Part print with two shaded views. Sizes in mm from the minimum x, y, z corner. A direction names the side the tool comes from. Round coordinates to 2 decimals unless told otherwise and drop trailing zeros. Order: outer loops, then holes, each group sorted by start corner. A loop starts at its lowest first (then second) coordinate and runs counter-clockwise, first axis right, second up. Notation, with made-up numbers: (46, -35.75) -> (53, -35.75) arc R32 ccw to (53, -5.75) -> close; hole circle Ø4 at (4, -14.75). An arc over 180 degrees is marked (long way). Put each result on its own line as item: value. Start each with the question number.
Q1. 3-axis set-ups, long thin cutter, end or side, ignore diameter. For the marked faces 4 and 5: which of +Z, -Z, +X, -X, +Y, -Y reach the whole face in a straight line?
Q2. Flat gauge pins, fed straight in: P1, Ø8, axis at x = 15.5, z = 28.5, coming from the +Y side; P2, Ø4.5, axis at y = 45, z = 10.5, coming from the -X side; P3, Ø20, axis at x = 40.5, y = 28, coming from the -Z side; P4, Ø1.9, axis at x = 29.19, y = 17.25, coming from the -Z side. Where does each tip first touch, or does it go through?
Q3. Probe L1, parallel to X at y = 47, z = 10; L2, parallel to Y at x = 61, z = 7; L3, parallel to Y at x = 17.5, z = 31.95. List the from-to ranges inside material, lowest first.
Q4. Pull direction Y, two halves, no side cores. Call the marked faces 1, 2 and 3: released by +Y, released by -Y, zero draft, split by the parting line, or undercut.
Q5. Cut at D-D, the plane y = 26. List the corners of the cut face in (x, z) (1 decimal).
Q6. Cut at B-B, the plane x = 92.5. List the corners of the cut face in (y, z), and give its area (3 significant figures).
Q7. Cut at A-A, the plane z = 15. List the corners of the cut face in (x, y).
Q8. Cut at C-C, the plane x = 81. List the corners of the cut face in (y, z).
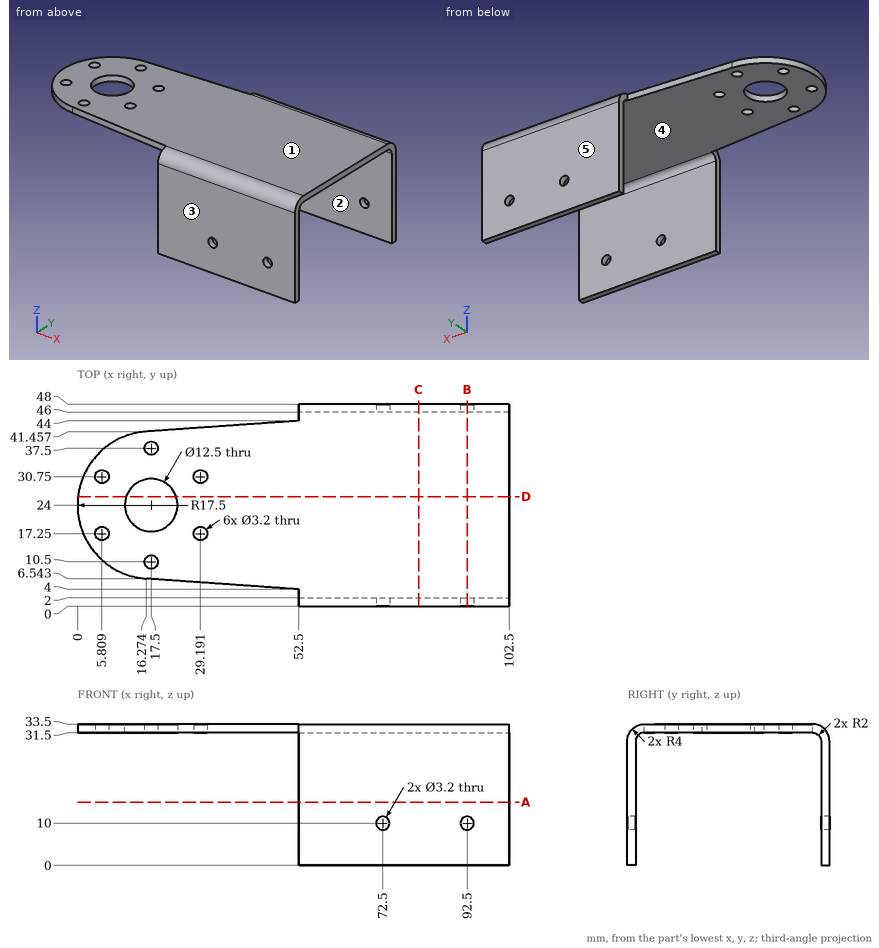
Ans:
1. face 4: -Z, +X, -X
1. face 5: +Z, -Z, +X, -X, +Y
2. P1: stops at y = 41.59
2. P2: stops at x = 52.5
2. P3: stops at z = 31.5
2. P4: passes through
3. L1: x = 52.5 to 70.9, 74.1 to 90.9, 94.1 to 102.5
3. L2: y = 0 to 2, 46 to 48
3. L3: y = 6.46 to 8.9, 12.1 to 17.75, 30.25 to 35.9, 39.1 to 41.54
4. face 1: zero draft
4. face 2: undercut
4. face 3: released by -Y
5. outline: (0.1, 31.5) -> (11.6, 31.5) -> (11.6, 33.5) -> (0.1, 33.5) -> close; (23.4, 31.5) -> (102.5, 31.5) -> (102.5, 33.5) -> (23.4, 33.5) -> close
6. outline: (0, 0) -> (2, 0) -> (2, 8.4) -> (0, 8.4) -> close; (0, 11.6) -> (2, 11.6) -> (2, 29.5) arc R2 cw to (4, 31.5) -> (44, 31.5) arc R2 cw to (46, 29.5) -> (46, 11.6) -> (48, 11.6) -> (48, 29.5) arc R4 ccw to (44, 33.5) -> (4, 33.5) arc R4 ccw to (0, 29.5) -> close; (46, 0) -> (48, 0) -> (48, 8.4) -> (46, 8.4) -> close
6. area: 204 mm^2
7. outline: (52.5, 0) -> (102.5, 0) -> (102.5, 2) -> (52.5, 2) -> close; (52.5, 46) -> (102.5, 46) -> (102.5, 48) -> (52.5, 48) -> close
8. outline: (0, 0) -> (2, 0) -> (2, 29.5) arc R2 cw to (4, 31.5) -> (44, 31.5) arc R2 cw to (46, 29.5) -> (46, 0) -> (48, 0) -> (48, 29.5) arc R4 ccw to (44, 33.5) -> (4, 33.5) arc R4 ccw to (0, 29.5) -> close
